Verification items for the finished model (mm, model axes). A direction names the side the tool comes from. Coordinates: 2 decimals unless noted, no trailing zeros. Loops run counter-clockwise (first coordinate to the right, second up) from the corner with the lowest first, then second, coordinate; pieces in that order, holes last. Notation, with made-up numbers: M 53.5,82 L 67.5,82 A31 ccw 67.5,114 Z; hole C -34.75,87.5 d8. An arc over 180 degrees is marked long. Write item = value, one per line. Start each with the question number.
Autodesk Inventor part; units mm, degrees
ref_plane "YZ Plane" through (0, 0, 0) normal (1, 0, 0) x (0, 1, 0)
ref_plane "XZ Plane" through (0, 0, 0) normal (0, 1, 0) x (-1, 0, 0)
ref_plane "XY Plane" through (0, 0, 0) normal (0, 0, 1) x (1, 0, 0)
sketch "Esquisse1" plane through (0, 0, 0) normal (0, 1, 0) x (-1, 0, 0)
  circle A0 centre (0, 0) radius 17.5
  circle A1 centre (0, 19.4) radius 1.75
  line L0 (13, 0) -> (-12, 0)
  circle A2 centre (0, -19.4) radius 1.75
  circle A3 centre (0, 19.4) radius 5.9464
  line L1 (4.7769, 22.9414) -> (14.0581, 10.422)
  line L2 (0, 31) -> (0, -30)
  line L3 (-4.7769, 22.9414) -> (-14.0581, 10.422)
  circle A4 centre (0, -19.4) radius 5.9464
  line L4 (4.7769, -22.9414) -> (14.0581, -10.422)
  line L5 (-4.7769, -22.9414) -> (-14.0581, -10.422)
  dimension "d1" = 35
  dimension "d3" = 11.8928
  dimension "d0" = 3.5
  dimension "d2" = 19.4
extrude "Extrusion1" add sketch "Esquisse1" along normal blind 2 contours A0 A4 L2 A3 | A0 A3 L1 | L4 A4 A0 | A3 L2 A0 | A0 L2 A1 A3 | A4 L2 A2 A0 | A0 L2 A4 | L2 A3 A0 | A0 A3 L2 A1 | L2 A4 A0 A3 | L2 A2 A4 A0 | A0 A4 L2 | A0 L3 A3 | A4 L5 A0
sketch "Esquisse2" plane through (0, 0, 0) normal (0, -1, 0) x (1, 0, 0)
  circle A0 centre (0, 0) radius 14.5602
extrude "Extrusion2" add sketch "Esquisse2" along normal blind 17
fillet "Congé1" radius 13.25 1 edges at (-14.5602, -17, 0)
properties part number "roulette"
Q1. Sectioned sample at B-B on x = 0. Count the separate pieces of the cut face and the enclosed holes in it, plus the area to 3 significant figures.
Q2. Sectioned sample at A-A on z = 19.4. Record the cut outline in (x, y), plus the area to 3 significant figures.
Q3. Gauge pin test, flat ends, axial feed: pin 1 (4 mm diameter, centred on x = 7.5, y = -14, fed in from +Z); pin 2 (2 mm diameter, centred on y = -0.5, z = -17.5, fed in from +X); pin 3 (4 mm diameter, centred on x = 3, y = -13, fed in from +Z). Record the tip position at first contact, or that the pin passes through.
Q4. Set-up check for faces 4 (the face through (0.078, 0.986, 25.346)), 5 (the face through (-6.4, 0, 13.3)): record each of +Z, -Z, +X, -X, +Y, -Y from which the full face is reachable in a straight line by a thin tool's end or side.
Q5. Scan lines: L1, parallel to Z at x = 0, y = 0.45; L2, parallel to Y at x = 2, z = -17; L3, parallel to X at y = 1.2, z = 19.4. Record each from-to range of solid material in increasing order. Write a range as [from, to].
Q6. Mould release check, pull along Z, two halves, no side actions. Record for faces 1 (the face through (-9.35, 0.99, -16.77)), 2 (the face through (-0.81, 0.99, 20.95)), 3 (the face through (-9.35, 0.99, 16.77)): +Z half, -Z half, draft (parallel to the pull), parting line (faces both ways), or undercut.
Solutions:
q1.separate_pieces = 3
q1.enclosed_holes = 0
q1.area = 507 mm²
q2.outline = M -7.4,0 L -1.75,0 L -1.75,2 L -7.4,2 Z; M 1.75,0 L 7.4,0 L 7.4,2 L 1.75,2 Z
q2.area = 22.6 mm²
q3.pin_1 = 9.44
q3.pin_2 = 9.45
q3.pin_3 = 12.1
q4.face_4 = +Z, +Y, -Y
q4.face_5 = -Y
q5.L1 = [-25.35, -21.15], [-17.65, 17.65], [21.15, 25.35]
q5.L2 = [0, 2]
q5.L3 = [-7.4, -1.75], [1.75, 7.4]
q6.face_1 = -Z half
q6.face_2 = undercut
q6.face_3 = +Z half
